Check sheet for the modelled part. Datum: model origin and axes. Units: mm. Face numbers are marked on the shaded views. A direction names the side the tool comes from. Give positions to 0.01 mm unless a question says otherwise; leave off trailing zeros. Order: outer loops, then holes, each group sorted by start corner. A loop starts at its lowest first (then second) coordinate and runs counter-clockwise, first axis right, second up. Notation, with made-up numbers: (6, 24.25) -> (65, 24.25) arc R11 cw to (65, 35.25) -> close; hole circle Ø2 at (-23, 43). An arc over 180 degrees is marked (long way). Answer in a Markdown table with one row per item. Add a question column.
(1) Set-up check for the marked faces 3, 4 and 5: record each of +Z, -Z, +X, -X, +Y, -Y from which the full face is reachable in a straight line by a thin tool's end or side.
(2) Thickness scan on L1, parallel to X at y = 8, z = 2; L2, parallel to X at y = -13.5, z = 1.75; L3, parallel to Y at x = -20.5, z = 3.75. Record the ranges inside material, lowest first. Write a range as [from, to].
(3) Cross-section at B-B (x = -12.5). Record the cut outline in (y, z).
(4) Go/stop test with flat-tipped pins: pin 1 (12 mm diameter, centred on x = 1, y = -9.5, fed in from +Z); pin 2 (1.8 mm diameter, centred on x = 23, y = 2, fed in from +Z); pin 3 (2.5 mm diameter, centred on x = 17, z = 3.5, fed in from +Y); pin 4 (3 mm diameter, centred on x = -16.5, y = -11.5, fed in from +Z). Record where each tip stops, or that it passes through.
(5) Release check for a two-part mould opening along X. For the marked faces 1 and 2 record: released by +X, released by -X, zero draft, split by the parting line, or undercut.
(6) Cross-section at C-C (y = 11). Record the cut outline in (x, z), then the cut area to 3 significant figures.
(7) Cross-section at A-A (y = -4). Record the cut outline in (x, z).
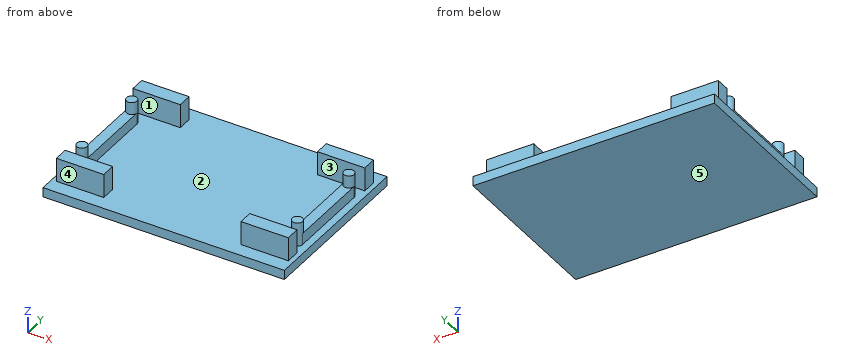
```python
from build123d import *

# Parameters (mm, degrees)
SKETCH030_W   = 51
SKETCH030_H   = 35.4
PAD011_DEPTH  = 2
SKETCH031_W   = 2.2
SKETCH031_H   = 17.18
SKETCH031_H_2 = 17.78
PAD012_DEPTH  = 2.4
SKETCH032_R   = 1.1
SKETCH032_W   = 10
SKETCH032_H   = 3.02
PAD013_DEPTH  = 5


with BuildPart() as part:
    # Sketch030 (on DatumPlane) → Pad011 (new body)
    with BuildSketch(Plane.XY):
        Rectangle(SKETCH030_W, SKETCH030_H)
    extrude(amount=-PAD011_DEPTH)

    # Sketch031 (on DatumPlane) → Pad012 (join)
    with BuildSketch(Plane.XY):
        with Locations((-22.86, 0)):
            Rectangle(SKETCH031_W, SKETCH031_H)
        with Locations((22.86, 0)):
            Rectangle(SKETCH031_W, SKETCH031_H_2)
    extrude(amount=PAD012_DEPTH)

    # Sketch032 (on DatumPlane) → Pad013 (join)
    with BuildSketch(Plane.XY):
        with Locations((-22.86, -8.59)):
            Circle(SKETCH032_R)
        with Locations((-22.86, 8.59)):
            Circle(SKETCH032_R)
        with Locations((22.86, 8.89)):
            Circle(SKETCH032_R)
        with Locations((22.86, -8.89)):
            Circle(SKETCH032_R)
        with Locations((-19.5, 13.19)):
            Rectangle(SKETCH032_W, SKETCH032_H)
        with Locations((19.5, 13.19)):
            Rectangle(SKETCH032_W, SKETCH032_H)
        with Locations((-19.5, -13.19)):
            Rectangle(SKETCH032_W, SKETCH032_H)
        with Locations((19.5, -13.19)):
            Rectangle(SKETCH032_W, SKETCH032_H)
    extrude(amount=PAD013_DEPTH)


solid = part.part
```
Answer below:
| question | item | result |
|---|---|---|
| 1 | face 3 | +Z, +X, -X |
| 1 | face 4 | +Z, +X, -X, -Y |
| 1 | face 5 | -Z, +X, -X, +Y, -Y |
| 2 | L1 | x = [-23.96, -21.76], [21.76, 23.96] |
| 2 | L2 | x = [-24.5, -14.5], [14.5, 24.5] |
| 2 | L3 | y = [-14.7, -11.68], [11.68, 14.7] |
| 3 | outline | (-17.7, -2) -> (17.7, -2) -> (17.7, 0) -> (-17.7, 0) -> close |
| 4 | pin 1 | stops at z = 0 |
| 4 | pin 2 | stops at z = 2.4 |
| 4 | pin 3 | stops at y = 14.7 |
| 4 | pin 4 | stops at z = 5 |
| 5 | face 1 | zero draft |
| 5 | face 2 | undercut |
| 6 | outline | (-25.5, -2) -> (25.5, -2) -> (25.5, 0) -> (-25.5, 0) -> close |
| 6 | area | 102 mm² |
| 7 | outline | (-25.5, -2) -> (25.5, -2) -> (25.5, 0) -> (23.96, 0) -> (23.96, 2.4) -> (21.76, 2.4) -> (21.76, 0) -> (-21.76, 0) -> (-21.76, 2.4) -> (-23.96, 2.4) -> (-23.96, 0) -> (-25.5, 0) -> close |
